Autodesk Inventor part; units mm, degrees
ref_plane "YZ Plane" through (0, 0, 0) normal (1, 0, 0) x (0, 1, 0)
ref_plane "XZ Plane" through (0, 0, 0) normal (0, 1, 0) x (-1, 0, 0)
ref_plane "XY Plane" through (0, 0, 0) normal (0, 0, 1) x (1, 0, 0)
sketch "Sketch1" plane through (0, 0, 0) normal (0, 1, 0) x (-1, 0, 0)
  circle A0 centre (0, 0) radius 15
  dimension "d0" = 30
extrude "Extrusion1" add sketch "Sketch1" along normal blind 2
sketch "Sketch2" plane through (0, 2, 0) normal (0, 1, 0) x (1, 0, 0)
  circle A0 centre (0, 0) radius 15
  circle A1 centre (0, 0) radius 13.5
  circle A2 centre (0, 0) radius 11.5
  line L0 (11.1081, 2.9764) -> (13.04, 3.4941)
  line L1 (0, 0) -> (13.5, 0) construction
  line L2 (11.1081, -2.9764) -> (13.04, -3.4941)
  line L3 (0, 0) -> (13.5, 0) construction
  line L4 (8.1317, 8.1317) -> (9.5459, 9.5459)
  line L5 (0, 0) -> (13.5, 0) construction
  line L6 (2.9764, 11.1081) -> (3.4941, 13.04)
  line L7 (0, 0) -> (13.5, 0) construction
  line L8 (-2.9764, 11.1081) -> (-3.4941, 13.04)
  circle A3 centre (0, 0) radius 15
  line L9 (-8.1317, 8.1317) -> (-9.5459, 9.5459)
  line L10 (0, 0) -> (13.5, 0) construction
  line L11 (-9.5459, 9.5459) -> (-8.1317, 8.1317)
  line L12 (8.1317, -8.1317) -> (9.5459, -9.5459)
  line L13 (-3.4941, 13.04) -> (-2.9764, 11.1081)
  line L14 (2.9764, -11.1081) -> (3.4941, -13.04)
  line L15 (9.5459, 9.5459) -> (8.1317, 8.1317)
  line L16 (-8.1317, -8.1317) -> (-9.5459, -9.5459)
  line L17 (3.4941, 13.04) -> (2.9764, 11.1081)
  line L18 (-2.9764, -11.1081) -> (-3.4941, -13.04)
  line L19 (13.04, 3.4941) -> (11.1081, 2.9764)
  line L20 (-11.1081, -2.9764) -> (-13.04, -3.4941)
  line L21 (13.04, -3.4941) -> (11.1081, -2.9764)
  line L22 (-11.1081, 2.9764) -> (-13.04, 3.4941)
extrude "Extrusion2" add sketch "Sketch2" along normal blind 4 contours L0 A2 L4 A1 | A1 L12 A2 L2 | L6 A2 L8 A1 | A1 L18 A2 L14 | L9 A2 L22 A1 | A1 L20 A2 L16
sketch "Sketch3" plane through (0, 2, 0) normal (0, 1, 0) x (1, 0, 0)
  line L0 (-2.9764, 11.1081) -> (-3.4941, 13.04)
  arc A0 (3.4941, 13.04) -> (-3.4941, 13.04) centre (0, 0) ccw
  line L1 (3.4941, 13.04) -> (2.9764, 11.1081)
  arc A1 (2.9764, 11.1081) -> (-2.9764, 11.1081) centre (0, 0) ccw
  line L2 (-3.4941, -13.04) -> (-2.9764, -11.1081)
  arc A2 (-2.9764, -11.1081) -> (2.9764, -11.1081) centre (0, 0) ccw
  line L3 (2.9764, -11.1081) -> (3.4941, -13.04)
  arc A3 (-3.4941, -13.04) -> (3.4941, -13.04) centre (0, 0) ccw
  line L4 (-11.1081, 2.9764) -> (-13.04, 3.4941)
  arc A4 (-9.5459, 9.5459) -> (-13.04, 3.4941) centre (0, 0) ccw
  line L5 (-9.5459, 9.5459) -> (-8.1317, 8.1317)
  arc A5 (-8.1317, 8.1317) -> (-11.1081, 2.9764) centre (0, 0) ccw
  line L6 (8.1317, 8.1317) -> (9.5459, 9.5459)
  arc A6 (13.04, 3.4941) -> (9.5459, 9.5459) centre (0, 0) ccw
  line L7 (13.04, 3.4941) -> (11.1081, 2.9764)
  arc A7 (11.1081, 2.9764) -> (8.1317, 8.1317) centre (0, 0) ccw
  line L8 (9.5459, -9.5459) -> (8.1317, -8.1317)
  arc A8 (8.1317, -8.1317) -> (11.1081, -2.9764) centre (0, 0) ccw
  line L9 (11.1081, -2.9764) -> (13.04, -3.4941)
  arc A9 (9.5459, -9.5459) -> (13.04, -3.4941) centre (0, 0) ccw
  line L10 (-13.04, -3.4941) -> (-11.1081, -2.9764)
  arc A10 (-11.1081, -2.9764) -> (-8.1317, -8.1317) centre (0, 0) ccw
  line L11 (-8.1317, -8.1317) -> (-9.5459, -9.5459)
  arc A11 (-13.04, -3.4941) -> (-9.5459, -9.5459) centre (0, 0) ccw
  circle A12 centre (0, 0) radius 15
  circle A13 centre (0, 0) radius 9.5
  dimension "d12" = 19
extrude "Extrusion3" add sketch "Sketch3" along normal blind 7 contours A13
sketch "Sketch4" plane through (0, 9, 0) normal (0, 1, 0) x (1, 0, 0)
  circle A0 centre (0, 0) radius 9.5
  circle A1 centre (0, 0) radius 7.5
  dimension "d15" = 15
extrude "Extrusion4" add sketch "Sketch4" along normal blind 2 contours A1
sketch "Sketch5" plane through (0, 0, 0) normal (0, -1, 0) x (1, 0, 0)
  circle A0 centre (0, 0) radius 7
  dimension "d18" = 14
extrude "Extrusion5" add sketch "Sketch5" along normal blind 7
properties part number "Bisagra final"
Check sheet for the modelled part. Datum: model origin and axes. Units: mm. A direction names the side the tool comes from. Coordinates: 2 decimals unless noted, no trailing zeros. Order: outer loops, then holes, each group sorted by start corner. A loop starts at its lowest first (then second) coordinate and runs counter-clockwise, first axis right, second up. Notation, with made-up numbers: (-23.75, 16) -> (23.25, 16) arc R30 ccw to (23.25, 39) -> close; hole circle Ø10 at (1.25, 74.5). An arc over 180 degrees is marked (long way). Write item = value, one per line. Start each with the question number.
1) Cross-section at D-D (y = -4). Enter the section's corners in (x, z), then the cut area to 3 significant figures.
2) Mould release check, pull along Z, two halves, no side actions. Record for faces 5 (the cylindrical face through (-11.716, 3.972, -6.707)), 6 (the flat face through (0, 6, -12)), 7 (the cylindrical face through (-7.493, 9.986, 0.33)), 8 (the cylindrical face through (-9.938, 3.972, 5.786)): +Z half, -Z half, draft (parallel to the pull), parting line (faces both ways), or undercut.
3) Access from +Z, -Z, +X, -X, +Y, -Y to the whole of each face (thin tool, end or side, straight path). Record for faces 1 (the cylindrical face through (0, 4, -11.5)), 2 (the cylindrical face through (6.466, -3.451, 2.681)), 3 (the flat face through (11, 6, -6)), 4 (the flat face through (3.23, 3.97, -12.06)).
4) Cross-section at A-A (y = 5.25). Enter the section's corners in (x, z), then the cut area to 3 significant figures.
5) Material ranges on L1, parallel to X at y = 2.5, z = -4; L2, parallel to Y at x = -7.75, z = -12.25; L3, parallel to Y at x = -11.75, z = -6, recorded low to high.
6) Go/stop test with flat-tipped pins: P1, Ø0.7, axis at x = -1, z = -12.5, coming from the +Y side; P2, Ø5.5, axis at x = 10.5, z = 4.5, coming from the +Y side; P3, Ø6, axis at x = 9.5, y = 0.5, coming from the -Z side. Record where each tip stops, or that it passes through.
7) Cross-section at B-B (x = 0). Enter the section's corners in (y, z), then the cut area to 3 significant figures.
8) Cross-section at C-C (z = 0). Enter the section's corners in (x, y).
Ans:
q1.outline = circle Ø14 at (0, 0)
q1.area = 154 mm²
q2.face_5 = -Z half
q2.face_6 = draft
q2.face_7 = parting line
q2.face_8 = undercut
q3.face_1 = +Y
q3.face_2 = -Y
q3.face_3 = -Z, +X, +Y
q3.face_4 = +X, +Y
q4.outline = (-13.04, -3.49) arc R13.5 ccw to (-9.55, -9.55) -> (-8.13, -8.13) arc R11.5 cw to (-11.11, -2.98) -> close; (-13.04, 3.49) -> (-11.11, 2.98) arc R11.5 cw to (-8.13, 8.13) -> (-9.55, 9.55) arc R13.5 ccw to start; circle Ø19 at (0, 0); (-3.49, -13.04) arc R13.5 ccw to (3.49, -13.04) -> (2.98, -11.11) arc R11.5 cw to (-2.98, -11.11) -> close; (-3.49, 13.04) -> (-2.98, 11.11) arc R11.5 cw to (2.98, 11.11) -> (3.49, 13.04) arc R13.5 ccw to start; (8.13, -8.13) -> (9.55, -9.55) arc R13.5 ccw to (13.04, -3.49) -> (11.11, -2.98) arc R11.5 cw to start; (8.13, 8.13) arc R11.5 cw to (11.11, 2.98) -> (13.04, 3.49) arc R13.5 ccw to (9.55, 9.55) -> close
q4.area = 362 mm²
q5.L1 = -12.89 to -10.78, -8.62 to 8.62, 10.78 to 12.89
q5.L2 = 0 to 2
q5.L3 = 0 to 6
q6.P1 = 6
q6.P2 = 9
q6.P3 = -13.52
q7.outline = (-7, -7) -> (0, -7) -> (0, -15) -> (2, -15) -> (2, -13.5) -> (6, -13.5) -> (6, -11.5) -> (2, -11.5) -> (2, -9.5) -> (9, -9.5) -> (9, -7.5) -> (11, -7.5) -> (11, 7.5) -> (9, 7.5) -> (9, 9.5) -> (2, 9.5) -> (2, 11.5) -> (6, 11.5) -> (6, 13.5) -> (2, 13.5) -> (2, 15) -> (0, 15) -> (0, 7) -> (-7, 7) -> close
q7.area = 337 mm²
q8.outline = (-15, 0) -> (-7, 0) -> (-7, -7) -> (7, -7) -> (7, 0) -> (15, 0) -> (15, 2) -> (9.5, 2) -> (9.5, 9) -> (7.5, 9) -> (7.5, 11) -> (-7.5, 11) -> (-7.5, 9) -> (-9.5, 9) -> (-9.5, 2) -> (-15, 2) -> close
